```python
from build123d import *

# Parameters (mm, degrees)
SKETCH1_R           = 7.5
BOSS_EXTRUDE1_DEPTH = 13
SKETCH3_R           = 5.8
CUT_EXTRUDE1_DEPTH  = 10
FILLET1_R           = 0.5


with BuildPart() as part:
    # Sketch1 → Boss-Extrude1 (new body)
    with BuildSketch(Plane.XY):
        with Locations(Location((0, 0, 0), (0, 0, 180))):
            Circle(SKETCH1_R)
    extrude(amount=BOSS_EXTRUDE1_DEPTH)

    # Sketch3 → Cut-Extrude1 (cut)
    with BuildSketch(Plane.XY.offset(13)):
        Circle(SKETCH3_R)
    extrude(amount=-CUT_EXTRUDE1_DEPTH, mode=Mode.SUBTRACT)

    # Fillet1
    fillet1_edges = [part.edges().sort_by_distance(p)[0] for p in [
        (7.5, 0, 0),
        (7.5, 0, 13),
        (-5.8, 0, 3),
        (-5.8, 0, 13),
    ]]
    fillet(fillet1_edges, radius=FILLET1_R)


solid = part.part
```
Source: CAD feature listing. Evaluate the final solid. Frame: model axes, mm. A direction names the side the tool comes from. Give positions to 0.01 mm unless a question says otherwise; leave off trailing zeros. Loops run counter-clockwise (first coordinate to the right, second up) from the corner with the lowest first, then second, coordinate; pieces in that order, holes last. Notation, with made-up numbers: (16, 29) - (34, 29) arc R16 cw to (34, 43) - close; hole circle Ø8 at (65, 3.25). An arc over 180 degrees is marked (long way). Use CSV: the item, a comma, the result in double quotes. Start each with the question number.
1. Reachability of faces 1 (the cylindrical face through (-5.794, 0.255, 8.063)), 2 (the flat face through (0, 0, 0)) from +Z, -Z, +X, -X, +Y, -Y: full face, straight path, thin tool, end or side. Return the list, or none.
2. Ray query, L1, parallel to Y at x = 0, z = 6.75; L2, parallel to Z at x = 4.5, y = 1.5; L3, parallel to X at y = 5, z = 6.25. Return the intervals inside material, ascending.
3. Draft query along X for faces 3 (the flat face through (6, -3, 13)), 4 (the cylindrical face through (-4.032, -6.324, 6.416)), 5 (the flat face through (0, 0, 3)). Return one class per face: +X half, -X half, draft (parallel to the pull), parting line (faces both ways), or undercut.
4. Section C-C (z = 8). Output: boundary loops of the cut face in (x, y).
5. Section A-A (y = 0). Output: boundary loops of the cut face in (x, z).
6. Pin query (flat end, axial travel): pin 1 (1 mm diameter, centred on x = 1.5, z = 11, fed in from -Y); pin 2 (5.5 mm diameter, centred on x = -1.5, y = -2, fed in from +Z); pin 3 (3 mm diameter, centred on x = 1, z = 4, fed in from -Y); pin 4 (1 mm diameter, centred on x = -2, z = 6, fed in from -Y). Return the tip coordinate at first contact, or that it passes through.
Response:
1,face 1,"+Z"
1,face 2,"-Z, +X, -X, +Y, -Y"
2,L1,"-7.5 to -5.8, 5.8 to 7.5"
2,L2,"0 to 3"
2,L3,"-5.59 to -2.94, 2.94 to 5.59"
3,face 3,"draft"
3,face 4,"parting line"
3,face 5,"undercut"
4,outline,"circle Ø15 at (0, 0); hole circle Ø11.6 at (0, 0)"
5,outline,"(-7.5, 0.5) arc R0.5 ccw to (-7, 0) - (7, 0) arc R0.5 ccw to (7.5, 0.5) - (7.5, 12.5) arc R0.5 ccw to (7, 13) - (6.3, 13) arc R0.5 ccw to (5.8, 12.5) - (5.8, 3.5) arc R0.5 cw to (5.3, 3) - (-5.3, 3) arc R0.5 cw to (-5.8, 3.5) - (-5.8, 12.5) arc R0.5 ccw to (-6.3, 13) - (-7, 13) arc R0.5 ccw to (-7.5, 12.5) - close"
6,pin 1,"y = -7.43"
6,pin 2,"z = 3"
6,pin 3,"y = -7.5"
6,pin 4,"y = -7.35"
